from build123d import *

# Parameters (mm, degrees)
SKETCH_1_W          = 192.3
SKETCH_1_H          = 144
SKETCH_1_R          = 1.75
EXTRUDE_1_DEPTH     = 4
SKETCH_2_W          = 100
SKETCH_2_H          = 90
CUT_EXTRUDE_1_DEPTH = 10
FILLET_1_R          = 10


with BuildPart() as part:
    # ｽｹｯﾁ1 → ﾎﾞｽ - 押し出し1 (new body)
    with BuildSketch(Plane.XY):
        Rectangle(SKETCH_1_W, SKETCH_1_H)
        with Locations((92.65, 67)):
            Circle(SKETCH_1_R, mode=Mode.SUBTRACT)
        with Locations((69.65, 67)):
            Circle(SKETCH_1_R, mode=Mode.SUBTRACT)
        with Locations((22.05, 67)):
            Circle(SKETCH_1_R, mode=Mode.SUBTRACT)
        with Locations((-0.95, 67)):
            Circle(SKETCH_1_R, mode=Mode.SUBTRACT)
        with Locations((-0.95, -67)):
            Circle(SKETCH_1_R, mode=Mode.SUBTRACT)
        with Locations((22.05, -67)):
            Circle(SKETCH_1_R, mode=Mode.SUBTRACT)
        with Locations((69.65, -67)):
            Circle(SKETCH_1_R, mode=Mode.SUBTRACT)
        with Locations((92.65, -67)):
            Circle(SKETCH_1_R, mode=Mode.SUBTRACT)
        with Locations((-90.15, 31.25)):
            Circle(SKETCH_1_R, mode=Mode.SUBTRACT)
        with Locations((-90.15, -31.25)):
            Circle(SKETCH_1_R, mode=Mode.SUBTRACT)
        with Locations((-58.15, 31.25)):
            Circle(SKETCH_1_R, mode=Mode.SUBTRACT)
        with Locations((-58.15, -31.25)):
            Circle(SKETCH_1_R, mode=Mode.SUBTRACT)
    extrude(amount=EXTRUDE_1_DEPTH)

    # ｽｹｯﾁ2 → ｶｯﾄ - 押し出し1 (cut)
    with BuildSketch(Plane.XY.offset(4)):
        with Locations((26.15, 0)):
            Rectangle(SKETCH_2_W, SKETCH_2_H)
    extrude(amount=-CUT_EXTRUDE_1_DEPTH, mode=Mode.SUBTRACT)

    # ﾌｨﾚｯﾄ1
    fillet_1_edges = [part.edges().sort_by_distance(p)[0] for p in [
        (-23.85, -45, 2),
        (-23.85, 45, 2),
        (76.15, 45, 2),
        (76.15, -45, 2),
    ]]
    fillet(fillet_1_edges, radius=FILLET_1_R)


solid = part.part
Here's how the part is built. I have some questions about the finished solid (model axes, mm). A direction names the side the tool comes from. Coordinates: 2 decimals unless noted, no trailing zeros. Write each loop counter-clockwise with the first axis right and the second up, starting at its lowest first coordinate (ties: lowest second). Pieces come first, ordered by that corner, then holes.
1) If we section it at A-A (x = 12): List the corners of the cut face in (y, z) for me.
Filled in:
outline: (-72, 0) - (-45, 0) - (-45, 4) - (-72, 4) - close; (45, 0) - (72, 0) - (72, 4) - (45, 4) - close
2) If we section it at B-B (z = 2.8): Count the separate pieces of the cut face and the enclosed holes in it, plus the area to 3 significant figures.
Filled in:
separate pieces: 1
enclosed holes: 13
area: 18,700 mm2
3) Thinking about a two-plate mould opening in Y: for faces 3 (the face through (76.15, 0, 2)), 4 (the face through (-20.84, 42.15, 1.97)), 5 (the face through (-1, 72, 2)), 6 (the face through (96.15, -1, 2)), which applies, +Y half, -Y half, draft (parallel to the pull), parting line (faces both ways), or undercut?
Filled in:
face 3: undercut
face 4: undercut
face 5: +Y half
face 6: draft
4) If I drill on line 1 (Y direction, x = 22, z = 2); line 2 (X direction, y = -67, z = 2.2); line 3 (Y direction, x = -90.15, z = 0.9), over which ranges is the centre line in solid material (lowest first)?
Filled in:
line 1: y = -72 to -68.75, -65.25 to -45, 45 to 65.25, 68.75 to 72
line 2: x = -96.15 to -2.7, 0.8 to 20.3, 23.8 to 67.9, 71.4 to 90.9, 94.4 to 96.15
line 3: y = -72 to -33, -29.5 to 29.5, 33 to 72
5) I'm going to push a flat-ended pin straight in: pin 1 (3 mm diameter, centred on x = 69.65, y = 67, fed in from -Z). Where does the tip first touch, or does it pass through?
Filled in:
pin 1: passes through
6) Which directions (+Z, -Z, +X, -X, +Y, -Y) give clear straight access to the entire face, cutting with the end or side of a thin tool? Please do faces 1 (the face through (73.14, -42.15, 1.97)), 2 (the face through (-1, -72, 2)).
Filled in:
face 1: +Z, -Z
face 2: +Z, -Z, +X, -X, -Y
7) If we section it at C-C (y = -24.5): List the corners of the cut face in (x, z) for me, plus the area to 3 significant figures.
Filled in:
outline: (-96.15, 0) - (-23.85, 0) - (-23.85, 4) - (-96.15, 4) - close; (76.15, 0) - (96.15, 0) - (96.15, 4) - (76.15, 4) - close
area: 369 mm2
